Autodesk Fusion 360 part; units mm, degrees
sketch "Esquisse1" plane through (0, 0, 0) normal (0, 0, 1) x (1, 0, 0)
  circle A0 centre (0, 0) radius 3.25
  dimension "d1" = 6.5
extrude "Extrusion1" add sketch "Esquisse1" along normal blind 1
sketch "Esquisse2" plane through (0, 0, 1) normal (0, 0, 1) x (-1, 0, 0)
  circle A0 centre (0, 0) radius 3.25
  line L0 (-0.45, 1.15) -> (0.45, 1.15)
  line L1 (0.45, 1.15) -> (0.45, -1.15)
  line L2 (0.45, -1.15) -> (-0.45, -1.15)
  line L3 (-0.45, -1.15) -> (-0.45, 1.15)
  line L4 (-0.45, 1.15) -> (0.45, -1.15) construction
  line L5 (0.45, 1.15) -> (-0.45, -1.15) construction
  dimension "d4" = 0.9
  dimension "d5" = 2.3
extrude "Extrusion2" add sketch "Esquisse2" along normal blind 3 contours L0 L1 L2 L3
Read the model definition and answer for the solid it produces. Units are mm, in the model's axes. A direction names the side the tool comes from. Coordinates: 2 decimals unless noted, no trailing zeros. Write each loop counter-clockwise with the first axis right and the second up, starting at its lowest first coordinate (ties: lowest second). Pieces come first, ordered by that corner, then holes. Notation, with made-up numbers: (19.25, 89) - (58.25, 89) arc R10 ccw to (58.25, 101) - close; hole circle Ø7 at (84.25, 26.25). An arc over 180 degrees is marked (long way). Answer as a JSON object with one key per item and string values. Group by question number.
1. Which of the six approach directions +Z, -Z, +X, -X, +Y, -Y give full straight-line access (tool end or side, diameter ignored) to faces 1 (the flat face through (0, 1.15, 2)), 2 (the flat face through (0, -1.15, 2)), 3 (the flat face through (0.45, 0, 2))?
2. Consider L1, parallel to Z at x = 1.75, y = 0.25; L2, parallel to X at y = 0.5, z = 1.85; L3, parallel to X at y = 2.75, z = 0.8. Determine where each line is inside the solid, lowest interval first. Write a range as [from, to].
3. A cutting plane is placed at D-D (y = 1.25). Determine the outline of the cut face in (x, z), plus the area to 3 significant figures.
4. A cutting plane is placed at C-C (z = 0.7). Determine the outline of the cut face in (x, y).
5. A cutting plane is placed at B-B (x = 0). Determine the outline of the cut face in (y, z), plus the area to 3 significant figures.
6. Each of these flat-tipped pins is pushed along its axis until it touches: P1, Ø2, axis at x = -2, z = 0.5, coming from the -Y side; P2, Ø1.5, axis at y = -0.5, z = 2, coming from the -X side. Where does it stop, or does it pass through?
7. A cutting plane is placed at A-A (y = 0). Determine the outline of the cut face in (x, z).
Worked out:
{
 "1": {"face 1": "+Z, +X, -X, +Y", "face 2": "+Z, +X, -X, -Y", "face 3": "+Z, +X, +Y, -Y"},
 "2": {"L1": "z = [0, 1]", "L2": "x = [-0.45, 0.45]", "L3": "x = [-1.73, 1.73]"},
 "3": {"outline": "(-3, 0) - (3, 0) - (3, 1) - (-3, 1) - close", "area": "6.00 mm²"},
 "4": {"outline": "circle Ø6.5 at (0, 0)"},
 "5": {"outline": "(-3.25, 0) - (3.25, 0) - (3.25, 1) - (1.15, 1) - (1.15, 4) - (-1.15, 4) - (-1.15, 1) - (-3.25, 1) - close", "area": "13.4 mm²"},
 "6": {"P1": "stops at y = -3.09", "P2": "stops at x = -0.45"},
 "7": {"outline": "(-3.25, 0) - (3.25, 0) - (3.25, 1) - (0.45, 1) - (0.45, 4) - (-0.45, 4) - (-0.45, 1) - (-3.25, 1) - close"}
}
